from build123d import *

# Parameters (mm, degrees)
F1_DEPTH = 762
F3_DEPTH = 762
F5_DEPTH = 2.778125


with BuildPart() as f1:
    # F0 (on Front) → F1 (new body)
    with BuildSketch(Plane.XZ):
        with BuildLine():
            Line((203.2, 355.6), (-203.2, 355.6))
            ThreePointArc((-203.2, 355.6), (-558.8, 0), (-203.2, -355.6))
            Line((-203.2, -355.6), (203.2, -355.6))
            ThreePointArc((203.2, -355.6), (558.8, 0), (203.2, 355.6))
        make_face()
    extrude(amount=F1_DEPTH)

    # F2 (on face) → F3 (cut, through all)
    with BuildSketch(Plane.XZ.offset(762)):
        with BuildLine():
            ThreePointArc((203.2, -352.821875), (556.021875, 0), (203.2, 352.821875))
            Line((203.2, 352.821875), (-203.2, 352.821875))
            ThreePointArc((-203.2, 352.821875), (-556.021875, 0), (-203.2, -352.821875))
            Line((-203.2, -352.821875), (203.2, -352.821875))
        make_face()
    extrude(amount=-F3_DEPTH, mode=Mode.SUBTRACT)

    # F4 (on face) → F5 (join)
    with BuildSketch(Plane.XZ.offset(762)):
        with BuildLine():
            ThreePointArc((-203.2, 355.6), (-558.8, 0), (-203.2, -355.6))
            Line((-203.2, -355.6), (203.2, -355.6))
            ThreePointArc((203.2, -355.6), (558.8, 0), (203.2, 355.6))
            Line((203.2, 355.6), (-203.2, 355.6))
        make_face()
        with BuildLine():
            ThreePointArc((203.2, 352.821875), (556.021875, 0), (203.2, -352.821875))
            Line((203.2, -352.821875), (-203.2, -352.821875))
            ThreePointArc((-203.2, -352.821875), (-556.021875, 0), (-203.2, 352.821875))
            Line((-203.2, 352.821875), (203.2, 352.821875))
        make_face(mode=Mode.SUBTRACT)
        with BuildLine():
            Line((-203.2, -352.821875), (203.2, -352.821875))
            ThreePointArc((203.2, -352.821875), (556.021875, 0), (203.2, 352.821875))
            Line((203.2, 352.821875), (-203.2, 352.821875))
            ThreePointArc((-203.2, 352.821875), (-556.021875, 0), (-203.2, -352.821875))
        make_face()
    extrude(amount=F5_DEPTH)

    # F6: F1 across plane


with BuildPart() as f1_1:
    add(f1.part)
    add(f1.part.mirror(Plane.XZ))


solid = f1_1.part
Read the model definition and answer for the solid it produces. Units are mm, in the model's axes. A direction names the side the tool comes from. Coordinates: 2 decimals unless noted, no trailing zeros. Loops run counter-clockwise (first coordinate to the right, second up) from the corner with the lowest first, then second, coordinate; pieces in that order, holes last. Notation, with made-up numbers: (45, 21) - (70, 21) arc R25 cw to (70, 59) - close; hole circle Ø10 at (52, 75). An arc over 180 degrees is marked (long way). Answer in a Markdown table with one row per item.
Q1. Given P1, Ø12, axis at y = -564.5, z = -87, coming from the -X side; P2, Ø2, axis at x = -277, y = -16, coming from the -Z side; P3, Ø4, axis at y = -445, z = -170, coming from the +X side, each flat-ended and moving along its own axis, determine where each tip first touches the part or whether it passes through.
Here are the results:
| item | result |
|---|---|
| P1 | stops at x = -549.45 |
| P2 | stops at z = -348.07 |
| P3 | stops at x = 516.61 |
Q2. The mould has two halves that part along Z. Classify faces 3 (the flat face through (-3, -11, -355.6)), 4 (the flat face through (-8, 762, 5)), 5 (the cylindrical face through (-558.714, -10.707, 7.819)): pulls with the +Z half, pulls with the -Z half, needs draft (parallel to the pull), parting line crosses it, or undercut.
Here are the results:
| item | result |
|---|---|
| face 3 | pulls with the -Z half |
| face 4 | undercut |
| face 5 | parting line crosses it |
Q3. Find section A-A on x = 144. Write down the section's boundary in (y, z), plus the area to 3 significant figures.
Here are the results:
| item | result |
|---|---|
| outline | (-764.78, -355.6) - (764.78, -355.6) - (764.78, 355.6) - (-764.78, 355.6) - close; hole (-762, -352.82) - (762, -352.82) - (762, 352.82) - (-762, 352.82) - close |
| area | 12,400 mm^2 |
Q4. Straight lines are drawn through the part: line 1 along Z through (x, y) = (178.5, 653.5); line 2 along Y through (x, z) = (-193, -146.5); line 3 along Z through (x, y) = (-212, -510.5). For each, find the intervals that lie inside material, in ascending order. Write a range as [from, to].
Here are the results:
| item | result |
|---|---|
| line 1 | z = [-355.6, -352.82], [352.82, 355.6] |
| line 2 | y = [-764.78, -762], [762, 764.78] |
| line 3 | z = [-355.49, -352.71], [352.71, 355.49] |
Q5. For faces 1 (the flat face through (3, -11, 355.6)), 2 (the cylindrical face through (-555.937, 10.668, 7.758)), determine the directions among +Z, -Z, +X, -X, +Y, -Y from which every point of the face is accessible in a straight line to the end or side of a thin tool.
Here are the results:
| item | result |
|---|---|
| face 1 | +Z, +X, -X, +Y, -Y |
| face 2 | none |
Q6. Find section B-B on y = -357. Write down the section's boundary in (x, z), plus the area to 3 significant figures.
Here are the results:
| item | result |
|---|---|
| outline | (-203.2, -355.6) - (203.2, -355.6) arc R355.6 ccw to (203.2, 355.6) - (-203.2, 355.6) arc R355.6 ccw to start; hole (-203.2, -352.82) - (203.2, -352.82) arc R352.82 ccw to (203.2, 352.82) - (-203.2, 352.82) arc R352.82 ccw to start |
| area | 8,440 mm^2 |
